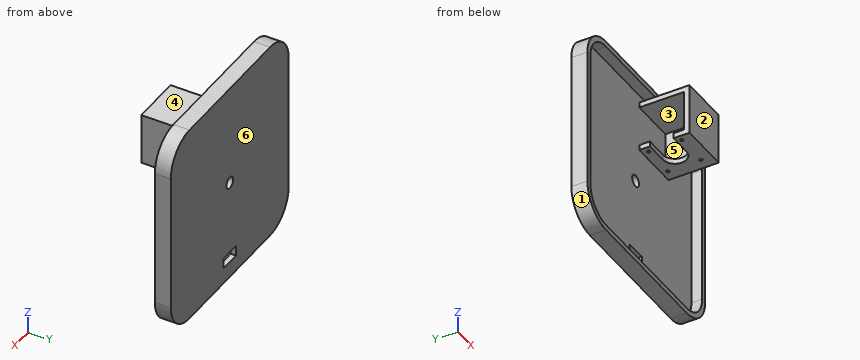
Autodesk Inventor part; units mm, degrees
ref_plane "YZ Plane" through (0, 0, 0) normal (1, 0, 0) x (0, 1, 0)
ref_plane "XZ Plane" through (0, 0, 0) normal (0, 1, 0) x (-1, 0, 0)
ref_plane "XY Plane" through (0, 0, 0) normal (0, 0, 1) x (1, 0, 0)
sketch "스케치1" plane through (0, 0, 0) normal (0, 1, 0) x (-1, 0, 0)
  line L0 (30, 0) -> (160, 0)
  line L1 (190, -30) -> (190, -160)
  line L2 (160, -190) -> (30, -190)
  line L3 (0, -160) -> (0, -30)
  arc A0 (190, -30) -> (160, 0) centre (160, -30) ccw
  arc A1 (160, -190) -> (190, -160) centre (160, -160) ccw
  arc A2 (0, -160) -> (30, -190) centre (30, -160) ccw
  arc A3 (30, 0) -> (0, -30) centre (30, -30) ccw
  point P0 (0, 0)
  point P1 (190, -190)
  point P2 (190, 0)
  point P3 (0, -190)
  dimension "d0" = 190
  dimension "d1" = 190
  dimension "d2" = 30
extrude "돌출1" add sketch "스케치1" along normal blind 15
shell "쉘1" thickness 5 removed faces 1 at (-106.6667, 0, -116.6667)
sketch "스케치3" plane through (0, 15, 0) normal (0, 1, 0) x (1, 0, 0)
  circle A0 centre (-95, 95) radius 5.5
  line L0 (-190, 160) -> (-190, 30)
  line L1 (-160, 0) -> (-30, 0)
  line L2 (-105, 175) -> (-85, 175)
  line L3 (-85, 175) -> (-85, 165)
  line L4 (-85, 165) -> (-105, 165)
  line L5 (-105, 165) -> (-105, 175)
  line L6 (-30, 190) -> (-160, 190)
  point P0 (0, 0)
  point P1 (-105, 170)
  dimension "d12" = 11
  dimension "d13" = 95
  dimension "d14" = 95
  dimension "d15" = 20
  dimension "d16" = 10
  dimension "d17" = 85
  dimension "d18" = 15
extrude "돌출3" cut sketch "스케치3" against normal blind 10
sketch "스케치4" plane through (-160, 10, -185) normal (0, -1, 0) x (1, 0, 0)
  circle A0 centre (65, 90) radius 22
  circle A1 centre (65, 90) radius 5.5
  line L0 (71, 130) -> (113, 130)
  line L1 (113, 130) -> (113, 125)
  line L2 (113, 125) -> (71, 125)
  line L3 (71, 125) -> (71, 130)
  line L4 (130, 0) -> (0, 0)
  line L5 (155, 155) -> (155, 25)
  line L6 (0, 180) -> (130, 180)
  line L7 (113, 125) -> (118, 125)
  line L8 (118, 125) -> (118, 163)
  line L9 (118, 163) -> (113, 163)
  line L10 (113, 163) -> (113, 125)
  point P0 (160, 185)
  point P1 (113, 127.5)
  point P2 (113, 130)
  dimension "d21" = 44
  dimension "d22" = 42
  dimension "d23" = 5
  dimension "d25" = 42
  dimension "d28" = 50
  dimension "d47" = 5
  dimension "d48" = 38
extrude "돌출4" add sketch "스케치4" along normal blind 42 contours L0 L1 L2 L3 | L10 L9 L8 L7 L1
sketch "스케치5" plane through (-47, 10, -60) normal (0, 0, -1) x (-1, 0, 0)
  circle A0 centre (5.5, -36.5) radius 1.5
  circle A1 centre (36.5, -36.5) radius 1.5
  circle A2 centre (36.5, -5.5) radius 1.5
  circle A3 centre (5.5, -5.5) radius 1.5
  line L0 (42, 0) -> (42, -42)
  line L1 (0, 0) -> (0, -42)
  line L2 (42, -42) -> (0, -42)
  circle A4 centre (21, -21) radius 11
  line L3 (21, -10) -> (42, -10)
  line L4 (42, -10) -> (42, -32)
  line L5 (42, -32) -> (21, -32)
  line L6 (21, -32) -> (21, -10)
  point P0 (-47, -10)
  point P1 (21, -32)
  dimension "d44" = 22
  dimension "d29" = 3
  dimension "d30" = 3
  dimension "d31" = 3
  dimension "d32" = 3
  dimension "d33" = 31
  dimension "d34" = 31
  dimension "d35" = 31
  dimension "d36" = 31
  dimension "d37" = 31
  dimension "d38" = 31
  dimension "d39" = 42
  dimension "d40" = 5.5
  dimension "d41" = 5.5
  dimension "d45" = 21
  dimension "d46" = 21
extrude "돌출5" cut sketch "스케치5" against normal blind 42
sketch "스케치6" plane through (-160, -32, -185) normal (0, -1, 0) x (1, 0, 0)
  line L0 (118, 163) -> (118, 125)
  line L1 (92, 125) -> (71, 125)
  line L2 (118, 163) -> (71, 163)
  line L3 (71, 163) -> (71, 125)
  line L4 (71, 125) -> (118, 125)
  line L5 (118, 125) -> (118, 163)
  point P0 (160, 185)
  point P1 (92, 125)
  point P2 (118, 125)
extrude "돌출6" add sketch "스케치6" along normal blind 5
sketch "스케치7" plane through (-47, 10, -22) normal (0, 0, 1) x (1, 0, 0)
  line L0 (0, 0) -> (5, 0)
  line L1 (0, 0) -> (0, -42)
  line L2 (0, -42) -> (-42, -42)
  line L3 (-42, -42) -> (-42, -47)
  line L4 (5, -47) -> (-42, -47)
  line L5 (5, 0) -> (5, -47)
  point P0 (47, -10)
extrude "돌출7" add sketch "스케치7" along normal blind 5
sketch "스케치8" plane through (-47, 10, -17) normal (0, 0, 1) x (1, 0, 0)
  line L0 (-42, -47) -> (5, -47)
  line L1 (5, -47) -> (5, 0)
  line L2 (-42, -47) -> (5, -47)
  line L3 (5, -47) -> (5, 0)
  line L4 (5, 0) -> (-42, 0)
  line L5 (-42, 0) -> (-42, -47)
  point P0 (47, -10)
extrude "돌출8" add sketch "스케치8" along normal blind 5
properties part number "top_3D 인쇄"
Design review of the part built by this model. Coordinates are the model's own, in mm. Face numbers are marked on the shaded views. A direction names the side the tool comes from. Give positions to 0.01 mm unless a question says otherwise; leave off trailing zeros. Loops run counter-clockwise (first coordinate to the right, second up) from the corner with the lowest first, then second, coordinate; pieces in that order, holes last. Notation, with made-up numbers: M 4,-18.5 L 8,-18.5 A16 ccw 8,2.5 Z; hole C -16.75,66 d8. An arc over 180 degrees is marked long. Return JSON: item names as keys, results as strings. Group by question number.
Item 1: We need section A-A (x = -95). Give the boundary of the cut face in (y, z).
Item 2: We need section B-B (y = -11). Give the boundary of the cut face in (x, z), and give its area (3 significant figures).
Item 3: Mouldability with a two-part tool opening along Z and no side actions: class the marked faces 1, 2 and 3 as released by +Z, released by -Z, zero draft, split by the parting line, or undercut.
Item 4: Insertion check: pin 1 Ø8 at (x, z) = (-50, -109.5) entering from -Y; pin 2 Ø1.5 at (y, z) = (-21.5, -29) entering from -X; pin 3 Ø2.5 at (y, z) = (12, -171) entering from -X. Each pin has a flat end and moves straight along its axis. Give the tip position at first contact, or say it passes through.
Item 5: For probe 1 along Y at (x, z) = (-83.5, -57.1); probe 2 along Z at (x, y) = (-68, 8.5); probe 3 along Z at (x, y) = (-67.5, -23), list the stretches that pass through material, from the lowest coordinate up.
Item 6: Tool access review of the marked faces 4, 5 and 6: name each direction out of +Z, -Z, +X, -X, +Y, -Y from which nothing blocks a thin tool from reaching the whole face with its end or side.
Item 7: We need section D-D (x = -65.5). Give the boundary of the cut face in (y, z).
Item 8: We need section C-C (z = -66.5). Give the boundary of the cut face in (x, y), and give its area (3 significant figures).
Output:
{
 "1": {"outline": "M 0,-190 L 15,-190 L 15,-175 L 10,-175 L 10,-185 L 0,-185 Z; M 0,-5 L 10,-5 L 10,-89.5 L 15,-89.5 L 15,0 L 0,0 Z; M 10,-165 L 15,-165 L 15,-100.5 L 10,-100.5 Z"},
 "2": {"outline": "M -89,-17 L -47,-17 L -47,-55 L -57,-55 L -57,-60 L -42,-60 L -42,-12 L -89,-12 Z", "area": "500 mm^2"},
 "3": {"face 1": "released by -Z", "face 2": "zero draft", "face 3": "undercut"},
 "4": {"pin 1": "stops at y = 10", "pin 2": "stops at x = -47", "pin 3": "stops at x = -188.37"},
 "5": {"probe 1": "y = -37 to -28, -25 to -22, 0 to 3, 6 to 15", "probe 2": "z = -190 to -185, -60 to -55, -17 to -12, -5 to 0", "probe 3": "z = -60 to -55, -17 to -12"},
 "6": {"face 4": "-Y", "face 5": "none", "face 6": "+Z, -Z, +X, -X, +Y"},
 "7": {"outline": "M -37,-60 L -21.71,-60 L -21.71,-55 L -32,-55 L -32,-17 L 10,-17 L 10,-55 L -0.29,-55 L -0.29,-60 L 10,-60 L 10,-185 L 0,-185 L 0,-190 L 15,-190 L 15,0 L 0,0 L 0,-5 L 10,-5 L 10,-12 L -37,-12 Z"},
 "8": {"outline": "M -190,0 L -185,0 L -185,10 L -5,10 L -5,0 L 0,0 L 0,15 L -190,15 Z", "area": "1,050 mm^2"}
}
